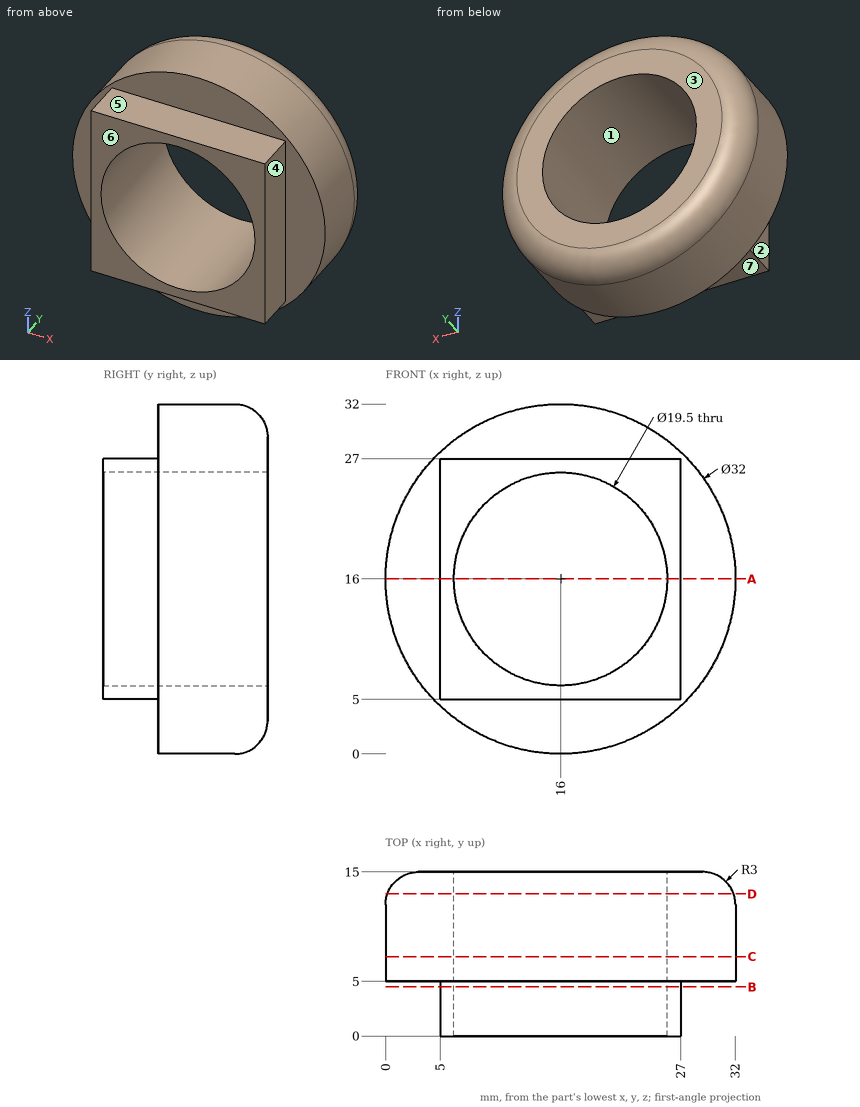
Part print with two shaded views. Sizes in mm from the minimum x, y, z corner. A direction names the side the tool comes from. Coordinates: 2 decimals unless noted, no trailing zeros. Write each loop counter-clockwise with the first axis right and the second up, starting at its lowest first coordinate (ties: lowest second). Pieces come first, ordered by that corner, then holes. Notation, with made-up numbers: (0.25, 14.5) - (38.25, 14.5) arc R18 ccw to (38.25, 48.5) - close; hole circle Ø3 at (76.5, -38.5). An arc over 180 degrees is marked (long way). One line per item, written item: value. Start each with the question number.
1. Slice it at D-D (y = 13). Write the cut outline in (x, z), plus the area to 3 significant figures.
2. Probe line 1 (X direction, y = 10.5, z = 16); line 2 (Y direction, x = 27.5, z = 13); line 3 (X direction, y = 13, z = 23.5). List the from-to ranges inside material, lowest first. Write a range as from..to.
3. Slice it at B-B (y = 4.5). Write the cut outline in (x, z), plus the area to 3 significant figures.
4. Tool access for the marked faces 5, 6 and 7: list every direction of +Z, -Z, +X, -X, +Y, -Y with a clear straight run to the whole face (end or side of a thin tool).
5. Mould opens along X. For the marked faces 1, 2, 3 and 4 say: released by +X, released by -X, zero draft, split by the parting line, or undercut.
6. Slice it at A-A (z = 16). Write the cut outline in (x, y).
7. Flat gauge pins, fed straight in: pin 1 (5 mm diameter, centred on y = 4, z = 12, fed in from -X); pin 2 (5 mm diameter, centred on x = 10.5, z = 21, fed in from +Y); pin 3 (2 mm diameter, centred on y = 8.5, z = 27.5, fed in from +X); pin 4 (5.5 mm diameter, centred on x = 11, y = 3, fed in from +Z). Where does each tip first touch, or does it go through?
8. Slice it at C-C (y = 7.25). Write the cut outline in (x, z), plus the area to 3 significant figures.
Answers below:
1. outline: circle Ø31.66 at (16, 16); hole circle Ø19.5 at (16, 16)
1. area: 488 mm^2
2. line 1: x = 0..6.25, 25.75..32
2. line 2: y = 5..15
2. line 3: x = 2.06..9.77, 22.23..29.94
3. outline: (5, 5) - (27, 5) - (27, 27) - (5, 27) - close; hole circle Ø19.5 at (16, 16)
3. area: 185 mm^2
4. face 5: +Z, +X, -X, -Y
4. face 6: +Z, -Z, +X, -X, -Y
4. face 7: -Z, +X, -X, -Y
5. face 1: undercut
5. face 2: released by -X
5. face 3: zero draft
5. face 4: released by +X
6. outline: (0, 5) - (5, 5) - (5, 0) - (6.25, 0) - (6.25, 15) - (3, 15) arc R3 ccw to (0, 12) - close; (25.75, 0) - (27, 0) - (27, 5) - (32, 5) - (32, 12) arc R3 ccw to (29, 15) - (25.75, 15) - close
7. pin 1: stops at x = 0.09
7. pin 2: stops at y = 15
7. pin 3: stops at x = 28.07
7. pin 4: stops at z = 31.69
8. outline: circle Ø32 at (16, 16); hole circle Ø19.5 at (16, 16)
8. area: 506 mm^2
